Check sheet for the modelled part. Datum: model origin and axes. Units: mm. A direction names the side the tool comes from. Round coordinates to 2 decimals unless told otherwise and drop trailing zeros. Write each loop counter-clockwise with the first axis right and the second up, starting at its lowest first coordinate (ties: lowest second). Pieces come first, ordered by that corner, then holes.
Item 1: Go/stop test with flat-tipped pins: pin 1 Ø1.5 at (y, z) = (2, 0.5) entering from +X; pin 2 Ø2 at (y, z) = (-3, -3) entering from -X. Record where each tip stops, or that it passes through.
Item 2: Material ranges on line 1 (Y direction, x = 0.75, z = 0.25); line 2 (X direction, y = 1.25, z = 4), recorded low to high.
Item 3: Tool access check on faces 1 (the cylindrical face through (4, 3.95, 0.08)), 2 (the flat face through (2, -1.1, 0)). Record the directions out of +Z, -Z, +X, -X, +Y, -Y that give a thin tool (end or side, any length) a straight path to the whole face; none if there is none.
Item 4: Cross-section at A-A on z = 0.5. Enter the section's corners in (x, y), plus the area to 3 significant figures.
Item 5: Cross-section at D-D on x = 4. Enter the section's corners in (y, z).
Item 6: Cross-section at C-C on x = 2. Enter the section's corners in (y, z).
Item 7: Cross-section at B-B on y = -0.5. Enter the section's corners in (x, z), plus the area to 3 significant figures.
Item 8: Release check for a two-part mould opening along Y. For faces 3 (the flat face through (-2, -1.1, 0)), 4 (the cylindrical face through (-4, 3.95, -0.08)), 5 (the cylindrical face through (3.95, -4, 0.08)), 6 (the flat face through (2, -2, -6)) record: +Y half, -Y half, draft (parallel to the pull), parting line (faces both ways), or undercut.
Autodesk Inventor part; units mm, degrees
ref_plane "YZ Plane" through (0, 0, 0) normal (1, 0, 0) x (0, 1, 0)
ref_plane "XZ Plane" through (0, 0, 0) normal (0, 1, 0) x (-1, 0, 0)
ref_plane "XY Plane" through (0, 0, 0) normal (0, 0, 1) x (1, 0, 0)
sketch "Boceto2" plane through (0, 0, 0) normal (0, 0, 1) x (1, 0, 0)
  circle A0 centre (0, 0) radius 1.6
  line L0 (1.1, -2.55) -> (-1.1, -2.55)
  line L1 (-1.1, -2.55) -> (-1.1, 2.55)
  line L2 (-1.1, 2.55) -> (1.1, 2.55)
  line L3 (1.1, 2.55) -> (1.1, -2.55)
  line L4 (1.1, -2.55) -> (-1.1, 2.55) construction
  line L5 (-1.1, -2.55) -> (1.1, 2.55) construction
  line L6 (-2.6, -1.1) -> (2.6, -1.1)
  line L7 (2.6, -1.1) -> (2.6, 1.1)
  line L8 (2.6, 1.1) -> (-2.6, 1.1)
  line L9 (-2.6, 1.1) -> (-2.6, -1.1)
  line L10 (-2.6, -1.1) -> (2.6, 1.1) construction
  line L11 (2.6, -1.1) -> (-2.6, 1.1) construction
  line L12 (5, -5) -> (-5, -5)
  line L13 (-5, -5) -> (-5, 5)
  line L14 (-5, 5) -> (5, 5)
  line L15 (5, 5) -> (5, -5)
  line L16 (5, -5) -> (-5, 5) construction
  line L17 (-5, -5) -> (5, 5) construction
  point P0 (-1.1, -1.1619)
  point P1 (-1.1619, -1.1)
  point P2 (-1.1619, 1.1)
  point P3 (-1.1, 1.1619)
  point P4 (1.1, 1.1619)
  point P5 (1.1619, 1.1)
  point P6 (1.1619, -1.1)
  point P7 (1.1, -1.1619)
  dimension "d0" = 3.2
  dimension "d1" = 2.2
  dimension "d2" = 5.1
  dimension "d3" = 2.2
  dimension "d4" = 5.2
  dimension "d5" = 10
  dimension "d6" = 10
extrude "Extrusión1" add sketch "Boceto2" along normal mid plane 12
fillet "Empalme1" radius 3.5 4 edges at (5, 5, 0) (-5, 5, 0) (5, -5, 0) (-5, -5, 0)
properties part number "Acoplador"
Response values:
1. pin 1: stops at x = 5
1. pin 2: stops at x = -4.96
2. line 1: y = -5 to -2.55, 2.55 to 5
2. line 2: x = -5 to -1.1, 1.1 to 5
3. face 1: +Z, -Z, +X, +Y
3. face 2: +Z, -Z
4. outline: (-5, -1.5) arc R3.5 ccw to (-1.5, -5) - (1.5, -5) arc R3.5 ccw to (5, -1.5) - (5, 1.5) arc R3.5 ccw to (1.5, 5) - (-1.5, 5) arc R3.5 ccw to (-5, 1.5) - close; hole (-2.6, -1.1) - (-1.16, -1.1) arc R1.6 ccw to (-1.1, -1.16) - (-1.1, -2.55) - (1.1, -2.55) - (1.1, -1.16) arc R1.6 ccw to (1.16, -1.1) - (2.6, -1.1) - (2.6, 1.1) - (1.16, 1.1) arc R1.6 ccw to (1.1, 1.16) - (1.1, 2.55) - (-1.1, 2.55) - (-1.1, 1.16) arc R1.6 ccw to (-1.16, 1.1) - (-2.6, 1.1) - close
4. area: 71.7 mm2
5. outline: (-3.95, -6) - (3.95, -6) - (3.95, 6) - (-3.95, 6) - close
6. outline: (-4.96, -6) - (-1.1, -6) - (-1.1, 6) - (-4.96, 6) - close; (1.1, -6) - (4.96, -6) - (4.96, 6) - (1.1, 6) - close
7. outline: (-5, -6) - (-2.6, -6) - (-2.6, 6) - (-5, 6) - close; (2.6, -6) - (5, -6) - (5, 6) - (2.6, 6) - close
7. area: 57.6 mm2
8. face 3: undercut
8. face 4: +Y half
8. face 5: -Y half
8. face 6: draft
